```python
from build123d import *

# Parameters (mm, degrees)
ESBO_O1_R                = 25
ESBO_O1_R_2              = 10
RESSALTO_EXTRUS_O1_DEPTH = 5
ESBO_O2_R                = 23
ESBO_O2_R_2              = 22.5
ESBO_O2_R_3              = 13.5
ESBO_O2_R_4              = 13
CORTE_EXTRUS_O1_DEPTH    = 0.25


with BuildPart() as part:
    # Esboço1 → Ressalto-extrusão1 (new, symmetric)
    with BuildSketch(Plane.XY):
        Circle(ESBO_O1_R)
        Circle(ESBO_O1_R_2, mode=Mode.SUBTRACT)
    extrude(amount=RESSALTO_EXTRUS_O1_DEPTH, both=True)

    # Esboço2 → Corte-extrusão1 (cut)
    # profile 1 of 2: a face of its own
    with BuildSketch(Plane.XY.offset(5)):
        Circle(ESBO_O2_R)
        Circle(ESBO_O2_R_2, mode=Mode.SUBTRACT)
    # profile 2 of 2: a face of its own
    with BuildSketch(Plane.XY.offset(5)):
        Circle(ESBO_O2_R_3)
        Circle(ESBO_O2_R_4, mode=Mode.SUBTRACT)
    corte_extrus_o1 = extrude(amount=-CORTE_EXTRUS_O1_DEPTH, mode=Mode.SUBTRACT)

    # Espelhar1: Corte-extrusão1 across plane
    add(corte_extrus_o1.mirror(Plane.XY), mode=Mode.SUBTRACT)


solid = part.part
```
Design review of the part built by this model. Coordinates are the model's own, in mm. A direction names the side the tool comes from. Round coordinates to 2 decimals unless told otherwise and drop trailing zeros. Write each loop counter-clockwise with the first axis right and the second up, starting at its lowest first coordinate (ties: lowest second). Pieces come first, ordered by that corner, then holes. Notation, with made-up numbers: (51, 88) -> (86, 88) arc R17 cw to (86, 105) -> close; hole circle Ø4 at (46.5, -17). An arc over 180 degrees is marked (long way). Write item = value, one per line. Start each with the question number.
1) Take a section at B-B, the plane y = 21.5. State the section outline as (x, z) points.
2) Take a section at A-A, the plane z = 1.75. State the section outline as (x, y) points, plus the area to 3 significant figures.
3) Clearance check with flat-ended pins moving along their axes: pin 1 (3 mm diameter, centred on x = 12, z = -4, fed in from +Y); pin 2 (4 mm diameter, centred on x = -11, z = -2.5, fed in from +Y); pin 3 (5 mm diameter, centred on y = 3.5, z = 1.5, fed in from +X). State where each tip first meets the part, or that it passes through.
4) Take a section at C-C, the plane y = -20.5. State the section outline as (x, z) points, plus the area to 3 significant figures.
5) Mouldability with a two-part tool opening along Y and no side actions: class faces 1 (the face through (23.846, 7.509, 0.07)), 2 (the face through (-7.1, 11.1, 4.75)), 3 (the face through (10, -10, -5)), 4 (the face through (-2.17, -9.76, -0.07)) as +Y half, -Y half, draft (parallel to the pull), parting line (faces both ways), or undercut.
6) Wall thickness on probe 1 along Y at (x, z) = (0, -4.8); probe 2 along Y at (x, z) = (-2, 2.75); probe 3 along Y at (x, z) = (-6, -3.25): over which ranges is each line inside the solid? List them lowest first. Write a range as from..to.
7) Tool access review of faces 5 (the face through (17, -15, 4.75)), 6 (the face through (17, -15, -4.75)), 7 (the face through (10, -10, 5)): name each direction out of +Z, -Z, +X, -X, +Y, -Y from which nothing blocks a thin tool from reaching the whole face with its end or side.
Results list:
q1.outline = (-12.76, -5) -> (-8.17, -5) -> (-8.17, -4.75) -> (-6.63, -4.75) -> (-6.63, -5) -> (6.63, -5) -> (6.63, -4.75) -> (8.17, -4.75) -> (8.17, -5) -> (12.76, -5) -> (12.76, 5) -> (8.17, 5) -> (8.17, 4.75) -> (6.63, 4.75) -> (6.63, 5) -> (-6.63, 5) -> (-6.63, 4.75) -> (-8.17, 4.75) -> (-8.17, 5) -> (-12.76, 5) -> close
q2.outline = circle Ø50 at (0, 0); hole circle Ø20 at (0, 0)
q2.area = 1,650 mm²
q3.pin_1 = 22.69
q3.pin_2 = 23.32
q3.pin_3 = 24.98
q4.outline = (-14.31, -5) -> (-10.43, -5) -> (-10.43, -4.75) -> (-9.27, -4.75) -> (-9.27, -5) -> (9.27, -5) -> (9.27, -4.75) -> (10.43, -4.75) -> (10.43, -5) -> (14.31, -5) -> (14.31, 5) -> (10.43, 5) -> (10.43, 4.75) -> (9.27, 4.75) -> (9.27, 5) -> (-9.27, 5) -> (-9.27, 4.75) -> (-10.43, 4.75) -> (-10.43, 5) -> (-14.31, 5) -> close
q4.area = 285 mm²
q5.face_1 = parting line
q5.face_2 = undercut
q5.face_3 = draft
q5.face_4 = undercut
q6.probe_1 = -25..-23, -22.5..-13.5, -13..-10, 10..13, 13.5..22.5, 23..25
q6.probe_2 = -24.92..-9.8, 9.8..24.92
q6.probe_3 = -24.27..-8, 8..24.27
q7.face_5 = +Z
q7.face_6 = -Z
q7.face_7 = +Z, +X, -X, +Y, -Y
